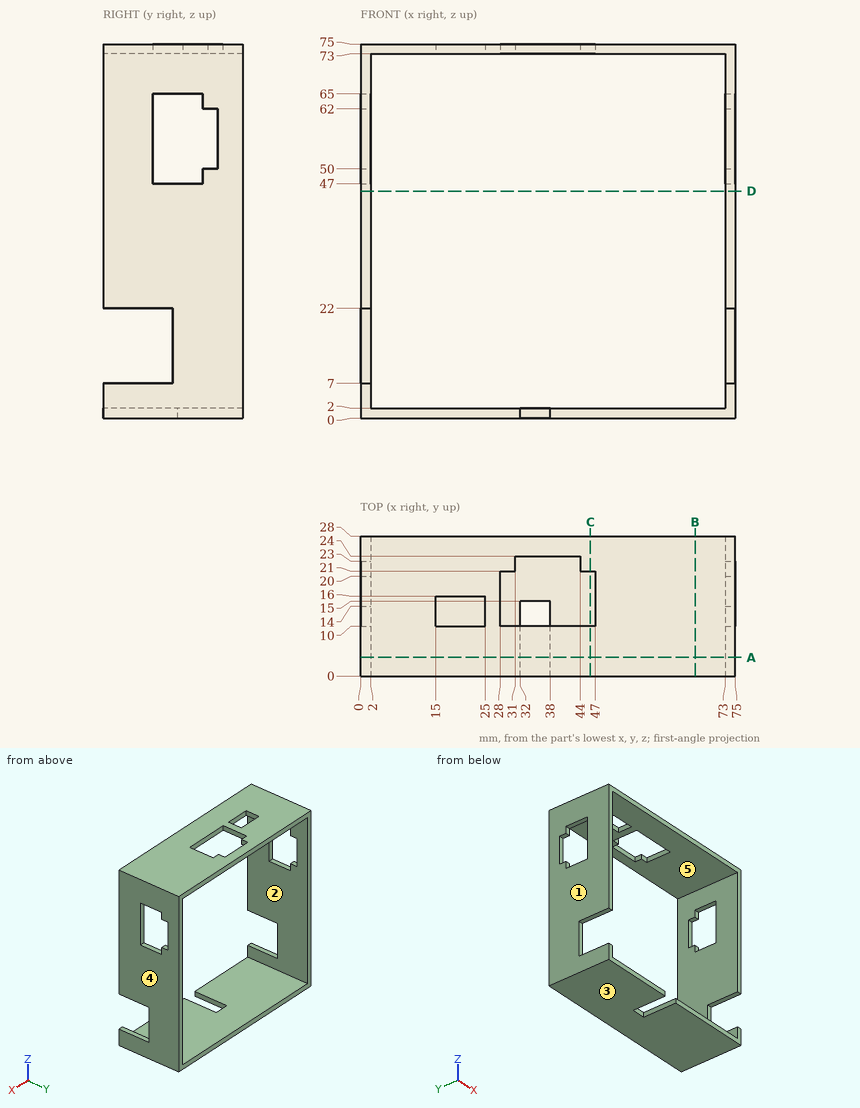
Study the drawing (mm; zero at the part's minimum x, y, z) and answer. A direction names the side the tool comes from. Give positions to 0.01 mm unless a question says otherwise; leave off trailing zeros. Order: outer loops, then holes, each group sorted by start corner. A loop starts at its lowest first (then second) coordinate and runs counter-clockwise, first axis right, second up. Notation, with made-up numbers: (85, 24.5) - (125, 24.5) arc R20 cw to (125, 28.5) - close; hole circle Ø10 at (5, 4). An arc over 180 degrees is marked (long way). Answer as CSV lines item,"result". Start each with the question number.
Q1. The mould has two halves that part along Z. Classify the marked faces 3, 4 and 5: +Z half, -Z half, draft (parallel to the pull), parting line (faces both ways), or undercut.
Q2. The part is cut by section A-A (y = 3.75). Write down the section's boundary in (x, z), then the cut area to 3 significant figures.
Q3. For the marked faces 1 and 2, determine the directions among +Z, -Z, +X, -X, +Y, -Y from which every point of the face is accessible in a straight line to the end or side of a thin tool.
Q4. The part is cut by section C-C (x = 46). Write down the section's boundary in (y, z).
Q5. The part is cut by section B-B (x = 67). Write down the section's boundary in (y, z).
Q6. Given pin 1 Ø5 at (y, z) = (25, 66.5) entering from -X; pin 2 Ø2 at (x, z) = (33.5, 1.5) entering from -Y, each flat-ended and moving along its own axis, determine where each tip first touches the part or whether it passes through.
Q7. Find the intervals of material crossed by L1, parallel to X at y = 10, z = 35.5, in increasing order. Write a range as [from, to].
Q8. The part is cut by section D-D (z = 45.5). Write down the section's boundary in (x, y), then the cut area to 3 significant figures.
Check result:
1,face 3,"-Z half"
1,face 4,"draft"
1,face 5,"undercut"
2,outline,"(0, 0) - (32, 0) - (32, 2) - (2, 2) - (2, 7) - (0, 7) - close; (0, 22) - (2, 22) - (2, 73) - (73, 73) - (73, 22) - (75, 22) - (75, 75) - (0, 75) - close; (38, 0) - (75, 0) - (75, 7) - (73, 7) - (73, 2) - (38, 2) - close"
2,area,"512 mm²"
3,face 1,"+Z, -Z, -X, +Y, -Y"
3,face 2,"+Y, -Y"
4,outline,"(0, 0) - (28, 0) - (28, 2) - (0, 2) - close; (0, 73) - (10, 73) - (10, 75) - (0, 75) - close; (21, 73) - (28, 73) - (28, 75) - (21, 75) - close"
5,outline,"(0, 0) - (28, 0) - (28, 2) - (0, 2) - close; (0, 73) - (28, 73) - (28, 75) - (0, 75) - close"
6,pin 1,"stops at x = 0"
6,pin 2,"stops at y = 15"
7,L1,"x = [0, 2], [73, 75]"
8,outline,"(0, 0) - (2, 0) - (2, 28) - (0, 28) - close; (73, 0) - (75, 0) - (75, 28) - (73, 28) - close"
8,area,"112 mm²"
